Part print with two shaded views. Sizes in mm from the minimum x, y, z corner. Round coordinates to 2 decimals unless told otherwise and drop trailing zeros. Loops run counter-clockwise (first coordinate to the right, second up) from the corner with the lowest first, then second, coordinate; pieces in that order, holes last. Notation, with made-up numbers: (79.25, 7.5) - (85.25, 7.5) arc R12 cw to (85.25, 26.5) - close; hole circle Ø3 at (29, 3). An arc over 180 degrees is marked (long way). Write each question's results on one line, items separated by ' | '. Start each with the question number.
(1) Cut at B-B, the plane y = 4. List the corners of the cut face in (x, z), then the cut area to 3 significant figures.
(2) Cut at C-C, the plane x = 33.5. List the corners of the cut face in (y, z), then the cut area to 3 significant figures.
(3) Drill centre lines: L1, parallel to Z at x = 127, y = 3; L2, parallel to Y at x = 163, z = 113.5; L3, parallel to X at y = 5.5, z = 130.5. Where is each one in solid material? Low to high.
(4) Flat gauge pins, fed straight in: P1, Ø3, axis at x = 249.17, z = 127, coming from the +Y side; P2, Ø12, axis at x = 48, z = 52.5, coming from the +Y side; P3, Ø1, axis at y = 14.5, z = 74.5, coming from the +X side. Where does each tip first touch, or does it go through?
(5) Cut at A-A, the plane z = 132.5. List the corners of the cut face in (x, y).
(6) Cut at D-D, the plane z = 166.5. List the corners of the cut face in (x, y), then the cut area to 3 significant figures.
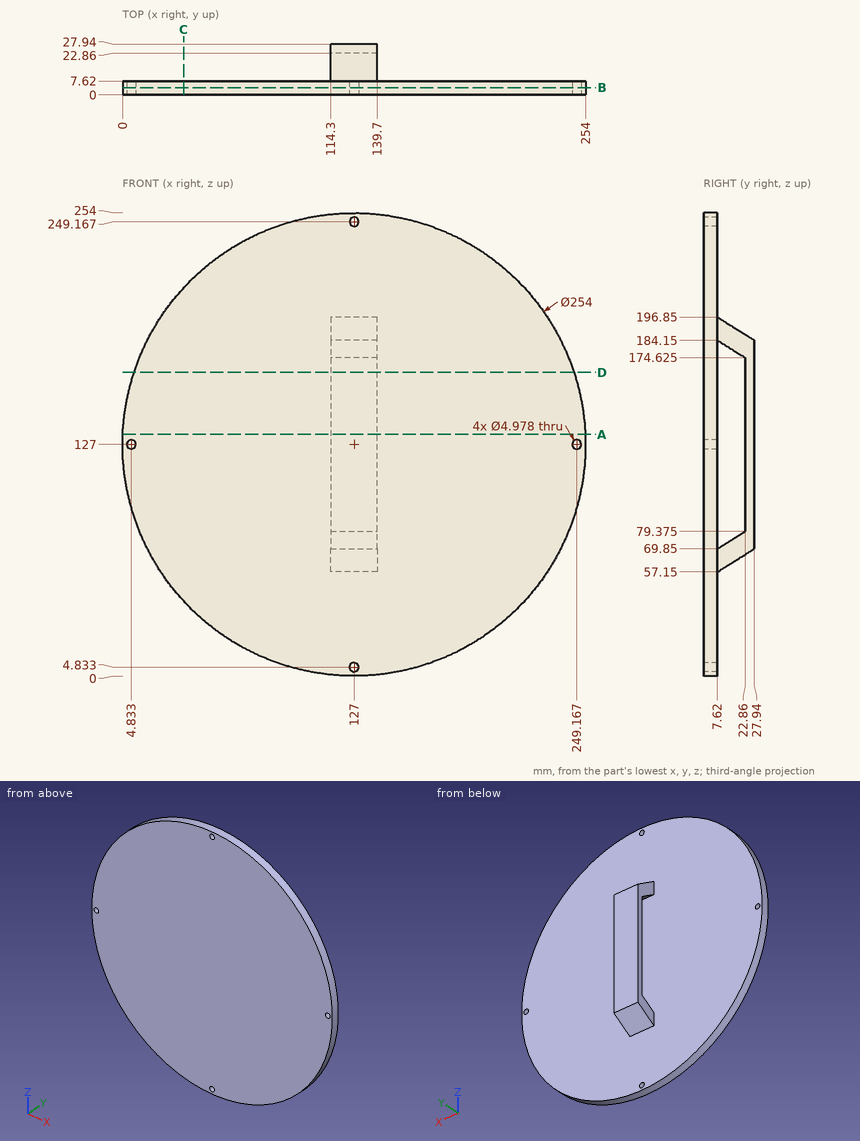
A:
1) outline: circle Ø254 at (127, 127); hole circle Ø4.98 at (4.83, 127); hole circle Ø4.98 at (127, 4.83); hole circle Ø4.98 at (127, 249.17); hole circle Ø4.98 at (249.17, 127) | area: 50,600 mm2
2) outline: (0, 41.05) - (7.62, 41.05) - (7.62, 212.95) - (0, 212.95) - close | area: 1,310 mm2
3) L1: 0 to 2.34, 7.32 to 246.68, 251.66 to 254 | L2: 0 to 7.62 | L3: 0.05 to 253.95
4) P1: through | P2: y = 7.62 | P3: x = 139.7
5) outline: (0.12, 0) - (253.88, 0) - (253.88, 7.62) - (0.12, 7.62) - close; (114.3, 22.86) - (139.7, 22.86) - (139.7, 27.94) - (114.3, 27.94) - close
6) outline: (6.3, 0) - (247.7, 0) - (247.7, 7.62) - (6.3, 7.62) - close; (114.3, 22.86) - (139.7, 22.86) - (139.7, 27.94) - (114.3, 27.94) - close | area: 1,970 mm2
